Design review of the part built by this model. Coordinates are the model's own, in mm. Face numbers are marked on the shaded views. A direction names the side the tool comes from. Coordinates: 2 decimals unless noted, no trailing zeros. Write each loop counter-clockwise with the first axis right and the second up, starting at its lowest first coordinate (ties: lowest second). Pieces come first, ordered by that corner, then holes. Notation, with made-up numbers: (66.5, -6.75) - (78.5, -6.75) arc R9 ccw to (78.5, 5.25) - close; hole circle Ø10 at (-10, 32.5). An arc over 180 degrees is marked (long way). Use a Markdown table: item, result.
from build123d import *

# Parameters (mm, degrees)
SKETCH_W           = 30
SKETCH_H           = 30
PAD_DEPTH          = 16
SKETCH001_R        = 7
PAD001_DEPTH       = 8
SKETCH002_R        = 4
POCKET_DEPTH       = 24
CYLINDER_R         = 6
CYLINDER_DEPTH     = 1
PAD002_DEPTH       = 7.25
SKETCH004_R        = 3.1
POCKET001_DEPTH    = 7
PAD003_DEPTH       = 7.25
SKETCH006_R        = 3.1
POCKET002_DEPTH    = 7
POCKET003_DEPTH    = 8
POLARPATTERN_COUNT = 4
FILLET_R           = 1
FILLET001_R        = 1.5
FILLET002_R        = 0.6


with BuildPart() as part:
    # Sketch → Pad (new body)
    with BuildSketch(Plane.XY):
        Rectangle(SKETCH_W, SKETCH_H)
    extrude(amount=PAD_DEPTH)

    # Sketch001 (on Face6 of Pad) → Pad001 (join)
    with BuildSketch(Plane.XY.offset(16)):
        Circle(SKETCH001_R)
    extrude(amount=PAD001_DEPTH)

    # Sketch002 (on Face8 of Pad001) → Pocket (cut)
    with BuildSketch(Plane.XY.offset(24)):
        Circle(SKETCH002_R)
    extrude(amount=-POCKET_DEPTH, mode=Mode.SUBTRACT)

    # Cylinder → Cylinder (cut)
    with BuildSketch(Plane.XY.offset(23)):
        Circle(CYLINDER_R)
    extrude(amount=CYLINDER_DEPTH, mode=Mode.SUBTRACT)

    # Sketch003 → Pad002 (join, symmetric)
    with BuildSketch(Plane.XZ):
        Polygon((15, 16), (22, 0), (22, -16), (15, -16), align=None)
    extrude(amount=PAD002_DEPTH, both=True)

    # Sketch004 (on Face16 of Pad002) → Pocket001 (cut)
    with BuildSketch(Plane(origin=(22, 0, 23), x_dir=(0, 1, 0), z_dir=(1, 0, 0))):
        with Locations((0, -32)):
            Circle(SKETCH004_R)
    extrude(amount=-POCKET001_DEPTH, mode=Mode.SUBTRACT)

    # Sketch005 → Pad003 (join, symmetric)
    with BuildSketch(Plane.YZ):
        Polygon((-15, 16), (-22, 0), (-22, -16), (-15, -16), align=None)
    extrude(amount=PAD003_DEPTH, both=True)

    # Sketch006 (on Face17 of Pad003) → Pocket002 (cut)
    with BuildSketch(Plane(origin=(0, -22, 23), x_dir=(1, 0, 0), z_dir=(0, -1, 0))):
        with Locations((0, -32)):
            Circle(SKETCH006_R)
    extrude(amount=-POCKET002_DEPTH, mode=Mode.SUBTRACT)

    # Sketch007 (on Face4 of Pocket002) → Pocket003 (cut)
    with BuildSketch(Plane(origin=(0, 0, 0), x_dir=(1, 0, 0), z_dir=(0, 0, -1))):
        with BuildLine():
            ThreePointArc((5.656854, 2), (4.242641, 4.242641), (2, 5.656854))
            Line((2, 13), (2, 5.656854))
            Line((2, 13), (13, 13))
            Line((13, 13), (13, 2))
            Line((13, 2), (5.656854, 2))
        make_face()
    pocket003 = extrude(amount=-POCKET003_DEPTH, mode=Mode.SUBTRACT)

    # PolarPattern: Pocket003 ×4 about axis
    polarpattern_axis = Axis((0, 0, 0), (0, 0, -1))
    for i in range(1, POLARPATTERN_COUNT):
        add(pocket003.rotate(polarpattern_axis, i * 360 / POLARPATTERN_COUNT), mode=Mode.SUBTRACT)

    # Fillet
    fillet_edges = [part.edges().sort_by_distance(p)[0] for p in [
        (5.656854, -2, 4),
        (2, -5.656854, 4),
        (2, -13, 4),
        (13, -13, 4),
        (13, -2, 4),
        (5.656854, 2, 4),
        (13, 2, 4),
        (13, 13, 4),
        (2, 13, 4),
        (2, 5.656854, 4),
        (-2, 5.656854, 4),
        (-13, 2, 4),
        (-13, 13, 4),
        (-2, 13, 4),
        (-5.656854, 2, 4),
        (-5.656854, -2, 4),
        (-2, -5.656854, 4),
        (-2, -13, 4),
        (-13, -13, 4),
        (-13, -2, 4),
    ]]
    fillet(fillet_edges, radius=FILLET_R)

    # Fillet001
    fillet001_edges = [part.edges().sort_by_distance(p)[0] for p in [
        (15, 15, 8),
        (-15, 15, 8),
        (-15, -15, 8),
        (15, -15, 8),
    ]]
    fillet(fillet001_edges, radius=FILLET001_R)

    # Fillet002
    fillet002_edges = [part.edges().sort_by_distance(p)[0] for p in [
        (18.5, -7.25, -16),
        (18.5, 7.25, -16),
        (7.25, -18.5, -16),
        (-7.25, -18.5, -16),
        (0, -22, -16),
        (0, -15, -16),
        (22, 0, -16),
        (15, 0, -16),
        (22, -7.25, -8),
        (15, -7.25, -8),
        (22, 7.25, -8),
        (15, 7.25, -8),
        (7.25, -15, -8),
        (7.25, -22, -8),
        (-7.25, -15, -8),
        (-7.25, -22, -8),
    ]]
    fillet(fillet002_edges, radius=FILLET002_R)


solid = part.part
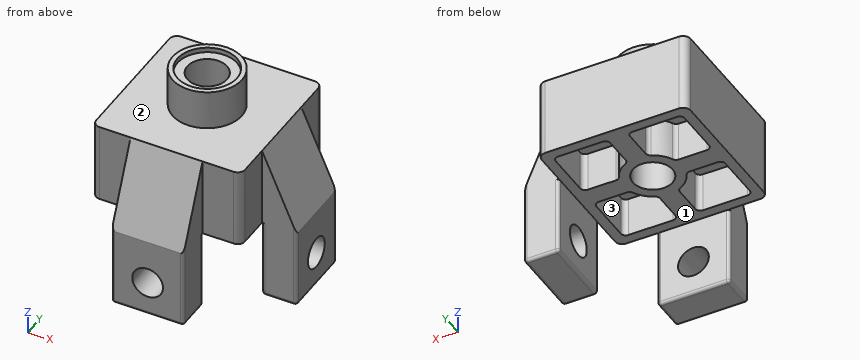
(1) Take a section at C-C on z = -9. Write out the cut boundary in (x, y), and give its area (3 significant figures).
Determined:
| item | result |
|---|---|
| outline | (-7.25, -21.4) arc R0.6 ccw to (-6.65, -22) - (-3.1, -22) - (-3.1, -15) - (-6.65, -15) arc R0.6 ccw to (-7.25, -15.6) - close; (3.1, -22) - (6.65, -22) arc R0.6 ccw to (7.25, -21.4) - (7.25, -15.6) arc R0.6 ccw to (6.65, -15) - (3.1, -15) - close; (15, -6.65) arc R0.6 ccw to (15.6, -7.25) - (21.4, -7.25) arc R0.6 ccw to (22, -6.65) - (22, -3.1) - (15, -3.1) - close; (15, 3.1) - (22, 3.1) - (22, 6.65) arc R0.6 ccw to (21.4, 7.25) - (15.6, 7.25) arc R0.6 ccw to (15, 6.65) - close |
| area | 116 mm2 |
(2) For pin 1 (1.5 mm diameter, centred on x = -2.5, z = 18.5, fed in from -Y); pin 2 (3.5 mm diameter, centred on x = 8, y = -7.5, fed in from -Z); pin 3 (5 mm diameter, centred on x = 12, z = 5, fed in from -Y), all flat-tipped, find the tip position at first contact; note any pin that passes through.
Determined:
| item | result |
|---|---|
| pin 1 | y = -6.78 |
| pin 2 | z = 8 |
| pin 3 | y = -15 |
(3) Take a section at A-A on x = 0. Write out the cut boundary in (y, z).
Determined:
| item | result |
|---|---|
| outline | (-22, -15.4) arc R0.6 ccw to (-21.4, -16) - (-15.6, -16) arc R0.6 ccw to (-15, -15.4) - (-15, -12.1) - (-22, -12.1) - close; (-22, -5.9) - (-15, -5.9) - (-15, 0) - (-4, 0) - (-4, 23) - (-6, 23) - (-6, 24) - (-7, 24) - (-7, 16) - (-15, 16) - (-22, 0) - close; (4, 0) - (15, 0) - (15, 16) - (7, 16) - (7, 24) - (6, 24) - (6, 23) - (4, 23) - close |
(4) For L1, parallel to Y at x = 3, z = 0.5; L2, parallel to Z at x = 0, y = -20.25; L3, parallel to Y at x = 0, z = 23.3, list the stretches that pass through material, from the lowest coordinate up. Write a range as from..to.
Determined:
| item | result |
|---|---|
| L1 | -21.78..-13, -5.2..-2.65, 2.65..5.2, 13..15 |
| L2 | -16..-12.1, -5.9..4 |
| L3 | -7..-6, 6..7 |
(5) Take a section at B-B on y = 0. Write out the cut boundary in (x, z).
Determined:
| item | result |
|---|---|
| outline | (-15, 0) - (-4, 0) - (-4, 23) - (-6, 23) - (-6, 24) - (-7, 24) - (-7, 16) - (-15, 16) - close; (4, 0) - (15, 0) - (15, -5.9) - (22, -5.9) - (22, 0) - (15, 16) - (7, 16) - (7, 24) - (6, 24) - (6, 23) - (4, 23) - close; (15, -15.4) arc R0.6 ccw to (15.6, -16) - (21.4, -16) arc R0.6 ccw to (22, -15.4) - (22, -12.1) - (15, -12.1) - close |
(6) Machinability: for the marked faces 1, 2 and 3, which of the approach directions +Z, -Z, +X, -X, +Y, -Y give a long, thin tool a straight path to every point of the face, cutting with its end or side? Answer none if there is none.
Determined:
| item | result |
|---|---|
| face 1 | -Z, -X, +Y |
| face 2 | +Z |
| face 3 | -Z |
(7) Take a section at D-D on y = -18.5. Write out the cut boundary in (x, z).
Determined:
| item | result |
|---|---|
| outline | (-7.25, -15.4) arc R0.6 ccw to (-6.65, -16) - (6.65, -16) arc R0.6 ccw to (7.25, -15.4) - (7.25, 8) - (-7.25, 8) - close; hole circle Ø6.2 at (0, -9) |
